Geometry: final body of the model. Coordinates: model frame, mm. Give positions to 0.01 mm unless a question says otherwise; leave off trailing zeros. Loops run counter-clockwise (first coordinate to the right, second up) from the corner with the lowest first, then second, coordinate; pieces in that order, holes last. Notation, with made-up numbers: M 16.5,-9 L 24.5,-9 A20 ccw 24.5,-2 Z; hole C 76.5,82.5 d1. An arc over 180 degrees is marked long. Put each result on its own line as item: value.
```python
from build123d import *

# Parameters (mm, degrees)
SKETCH1_W           = 76.2
SKETCH1_H           = 101.6
BOSS_EXTRUDE1_DEPTH = 19.05
SKETCH3_R           = 3.81
CUT_EXTRUDE2_DEPTH  = 77.2
SKETCH6_R           = 3.81
CUT_EXTRUDE5_DEPTH  = 77.2
SKETCH5_R           = 5.08
CUT_EXTRUDE4_DEPTH  = 20.05
CHAMFER1_SIZE       = 2.54


with BuildPart() as part:
    # Sketch1 → Boss-Extrude1 (new body)
    with BuildSketch(Plane(origin=(0, 0, 0), x_dir=(0, 0, -1), z_dir=(1, 0, 0))):
        with Locations((38.1, 50.8)):
            Rectangle(SKETCH1_W, SKETCH1_H)
    extrude(amount=BOSS_EXTRUDE1_DEPTH)

    # Sketch3 → Cut-Extrude2 (cut, through all)
    with BuildSketch(Plane.XY):
        with Locations((9.525, 12.7)):
            Circle(SKETCH3_R)
    extrude(amount=-CUT_EXTRUDE2_DEPTH, mode=Mode.SUBTRACT)

    # Sketch6 → Cut-Extrude5 (cut, through all)
    with BuildSketch(Plane.XY):
        with Locations((9.525, 88.9)):
            Circle(SKETCH6_R)
    extrude(amount=-CUT_EXTRUDE5_DEPTH, mode=Mode.SUBTRACT)

    # Sketch5 → Cut-Extrude4 (cut, through all)
    with BuildSketch(Plane(origin=(19.05, 0, 0), x_dir=(0, 0, -1), z_dir=(1, 0, 0))):
        with Locations((38.1, 50.8)):
            Circle(SKETCH5_R)
    extrude(amount=-CUT_EXTRUDE4_DEPTH, mode=Mode.SUBTRACT)

    # Chamfer1
    chamfer1_edges = [part.edges().sort_by_distance(p)[0] for p in [
        (9.525, 0, 0),
        (9.525, 101.6, 0),
        (9.525, 101.6, -76.2),
        (9.525, 0, -76.2),
    ]]
    chamfer(chamfer1_edges, length=CHAMFER1_SIZE)


solid = part.part
```
Item 1: Mould query, pull axis X, two halves, no side actions, for faces 1 (the flat face through (0, 52, -46)), 2 (the flat face through (9, 50, 0)), 3 (the cylindrical face through (6.717, 91.475, -37.567)). Classes: pulls with the +X half, pulls with the -X half, needs draft (parallel to the pull), parting line crosses it, or undercut.
Output values:
face 1: pulls with the -X half
face 2: needs draft
face 3: undercut
Item 2: Section B-B on y = 12.7. Output: boundary loops of the cut face in (x, z) (3 decimals).
Output values:
outline: M 0,-76.2 L 5.715,-76.2 L 5.715,0 L 0,0 Z; M 13.335,-76.2 L 19.05,-76.2 L 19.05,0 L 13.335,0 Z
Item 3: Section A-A on z = -38.1. Output: boundary loops of the cut face in (x, y) (3 decimals), then the cut area to 3 significant figures.
Output values:
outline: M 0,0 L 19.05,0 L 19.05,45.72 L 0,45.72 Z; M 0,55.88 L 19.05,55.88 L 19.05,101.6 L 0,101.6 Z; hole C 9.525,12.7 d7.62; hole C 9.525,88.9 d7.62
area: 1,650 mm²
Item 4: Section D-D on y = 50.8. Output: boundary loops of the cut face in (x, z).
Output values:
outline: M 0,-76.2 L 19.05,-76.2 L 19.05,-43.18 L 0,-43.18 Z; M 0,-33.02 L 19.05,-33.02 L 19.05,0 L 0,0 Z
Item 5: Line query: probe 1 along Y at (x, z) = (9.5, -24); probe 2 along Y at (x, z) = (11.25, -54); probe 3 along Y at (x, z) = (6.5, -38.1). Output: solid intervals per line, ascending. Write a range as [from, to].
Output values:
probe 1: [0, 8.89], [16.51, 85.09], [92.71, 101.6]
probe 2: [0, 9.3], [16.1, 85.5], [92.3, 101.6]
probe 3: [0, 10.38], [15.02, 45.72], [55.88, 86.58], [91.22, 101.6]
Item 6: Section C-C on z = -51.5. Output: boundary loops of the cut face in (x, y) (3 decimals).
Output values:
outline: M 0,0 L 19.05,0 L 19.05,101.6 L 0,101.6 Z; hole C 9.525,12.7 d7.62; hole C 9.525,88.9 d7.62
